Read the model definition and answer for the solid it produces. Units are mm, in the model's axes. Coordinates: 2 decimals unless noted, no trailing zeros. Order: outer loops, then holes, each group sorted by start corner. A loop starts at its lowest first (then second) coordinate and runs counter-clockwise, first axis right, second up. Notation, with made-up numbers: M 43,0 L 84,0 A22 ccw 84,14 Z; hole C 53.5,63 d11. An arc over 180 degrees is marked long. Write each question's results on one line, items separated by ' | '.
```python
from build123d import *

# Parameters (mm, degrees)
F1_DEPTH = 3.175
F2_R     = 5.08
F3_R     = 5.08


# Not quite as in the source:
# - two fillets or chamfers of one size are made in one step


with BuildPart() as f1:
    # F0 (on Top) → F1 (new body)
    with BuildSketch(Plane.XY):
        Polygon((0, -34.215349704), (-53.7331599414, 0), (-75.9016672165, 14.1161106039), (-101.0106563997, 14.1161106039), (-101.0106563997, 7.5655808932), (-101.0106563997, 0), (-101.0106563997, -16.8134532869), (-74.3406563997, -16.8134532869), (-74.3406563997, -43.2344191068), (-74.3406563997, -119.4344191068), (-74.3406563997, -146.9356715679), (0, -183.8173121214), align=None)
        Polygon((53.7331599414, 0), (0, -34.215349704), (0, -183.8173121214), (74.3406563997, -146.9356715679), (74.3406563997, -119.4344191068), (74.3406563997, -43.2344191068), (74.3406563997, -16.8134532869), (101.0106563997, -16.8134532869), (101.0106563997, 14.1161106039), (75.9016672165, 14.1161106039), align=None)
    extrude(amount=F1_DEPTH)

    # F2
    f2_edges = [f1.edges().sort_by_distance(p)[0] for p in [
        (0, -34.21535, 1.5875),
    ]]
    fillet(f2_edges, radius=F2_R)

    # F3
    f3_edges = [f1.edges().sort_by_distance(p)[0] for p in [
        (-74.340656, -146.935672, 1.5875),
        (0, -183.817312, 1.5875),
        (74.340656, -146.935672, 1.5875),
        (-75.901667, 14.116111, 1.5875),
        (-101.010656, 14.116111, 1.5875),
        (75.901667, 14.116111, 1.5875),
        (-101.010656, -16.813453, 1.5875),
        (101.010656, 14.116111, 1.5875),
        (101.010656, -16.813453, 1.5875),
    ]]
    fillet(f3_edges, radius=F3_R)


solid = f1.part
```
(1) The part is cut by section A-A, the plane y = -27. Write down the section's boundary in (x, z) (3 decimals), then the cut area to 3 significant figures.
Conclusion:
outline: M -74.341,0 L -11.331,0 L -11.331,3.175 L -74.341,3.175 Z; M 11.331,0 L 74.341,0 L 74.341,3.175 L 11.331,3.175 Z | area: 400 mm²
(2) Given pin 1 (1 mm diameter, centred on x = 80.5, z = 2.5, fed in from -Y); pin 2 (1.5 mm diameter, centred on y = -90, z = 0.5, fed in from +X); pin 3 (1 mm diameter, centred on y = -101.5, z = 1.5, fed in from -X), each flat-ended and moving along its own axis, determine where each tip first touches the part or whether it passes through.
Conclusion:
pin 1: y = -16.81 | pin 2: x = 74.34 | pin 3: x = -74.34
(3) The part is cut by section C-C, the plane y = -107. Write down the section's boundary in (x, z) (3 decimals), then the cut area to 3 significant figures.
Conclusion:
outline: M -74.341,0 L 74.341,0 L 74.341,3.175 L -74.341,3.175 Z | area: 472 mm²
(4) The part is cut by section D-D, the plane x = -7. Write down the section's boundary in (y, z) (1 decimal).
Conclusion:
outline: M -180.3,0 L -29.8,0 L -29.8,3.2 L -180.3,3.2 Z
(5) The part is cut by section B-B, the plane z = 0.6. Write down the section's boundary in (x, y), then the cut area to 3 significant figures.
Conclusion:
outline: M -101.01,-11.73 A5.08 ccw -95.93,-16.81 L -74.34,-16.81 L -74.34,-143.79 A5.08 ccw -71.52,-148.34 L -2.26,-182.7 A5.08 ccw 2.26,-182.7 L 71.52,-148.34 A5.08 ccw 74.34,-143.79 L 74.34,-16.81 L 95.93,-16.81 A5.08 ccw 101.01,-11.73 L 101.01,9.04 A5.08 ccw 95.93,14.12 L 77.38,14.12 A5.08 ccw 74.65,13.32 L 2.73,-32.48 A5.08 cw -2.73,-32.48 L -74.65,13.32 A5.08 ccw -77.38,14.12 L -95.93,14.12 A5.08 ccw -101.01,9.04 Z | area: 24,600 mm²
(6) Straight lines are drawn through the part: line 1 (Y direction, x = 80, z = 2.5); line 2 (X direction, y = -63, z = 1); line 3 (X direction, y = -32.5, z = 1.45). For each, find the intervals that lie inside material, in ascending order.
Conclusion:
line 1: -16.81 to 14.12 | line 2: -74.34 to 74.34 | line 3: -74.34 to -2.69, 2.69 to 74.34
